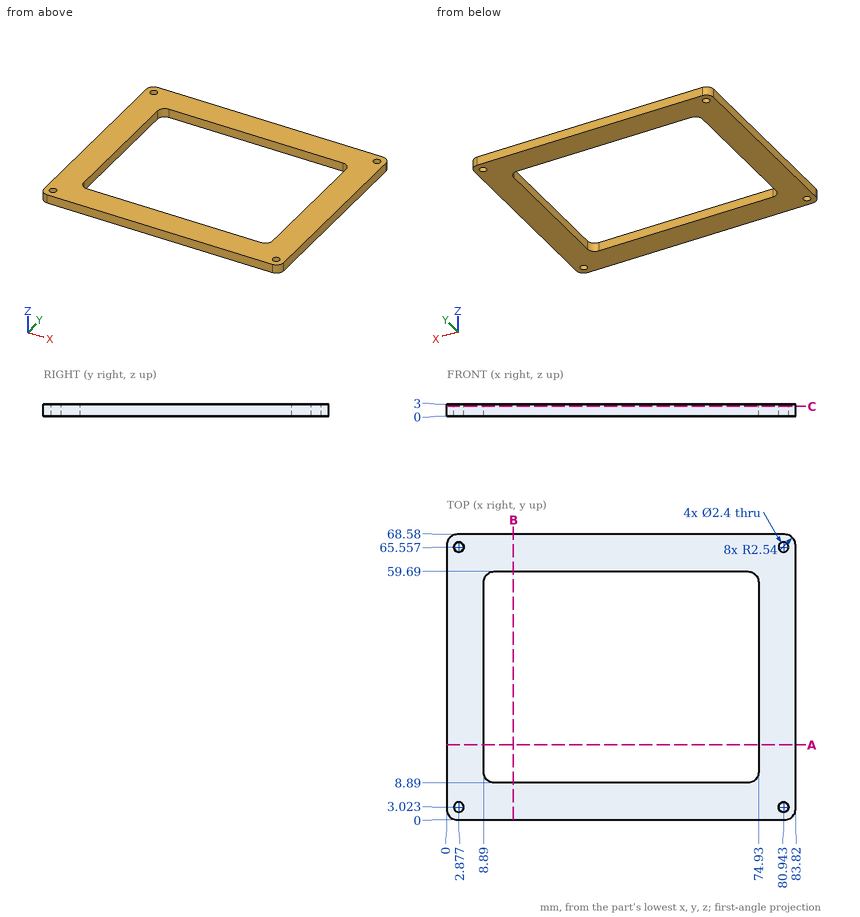
For this review, use the dimensioned drawing (mm, ordinates from the lowest corner) and the shaded views. Give positions to 0.01 mm unless a question says otherwise; leave off trailing zeros. Order: outer loops, then holes, each group sorted by start corner. A loop starts at its lowest first (then second) coordinate and runs counter-clockwise, first axis right, second up. Notation, with made-up numbers: M -21,44 L 32,44 A13 ccw 32,67 Z; hole C 18.5,-11.5 d1. An arc over 180 degrees is marked long. One line per question, with ' | ' between items. Start each with the question number.
1) Consider section C-C, the plane z = 2.4. Give the boundary of the cut face in (x, y).
2) Consider section B-B, the plane x = 16. Give the boundary of the cut face in (y, z).
3) Wall thickness on L1, parallel to X at y = 24.5, z = 2.8; L2, parallel to Y at x = 46, z = 1.4; L3, parallel to X at y = 64.5, z = 1.75 (1 decimal): over which ranges is each line inside the solid? List them lowest first. Write a range as from..to.
4) Consider section A-A, the plane y = 18. Give the boundary of the cut face in (x, z).
5) Clearance check with a flat-ended pin moving along its axis: P1, Ø2, axis at x = 80.94, y = 65.56, coming from the -Z side. State where the tip first meets the part, or that it passes through.
Found:
1) outline: M 0,2.54 A2.54 ccw 2.54,0 L 81.28,0 A2.54 ccw 83.82,2.54 L 83.82,66.04 A2.54 ccw 81.28,68.58 L 2.54,68.58 A2.54 ccw 0,66.04 Z; hole C 2.88,3.02 d2.4; hole C 2.88,65.56 d2.4; hole M 8.89,11.43 A2.54 ccw 11.43,8.89 L 72.39,8.89 A2.54 ccw 74.93,11.43 L 74.93,57.15 A2.54 ccw 72.39,59.69 L 11.43,59.69 A2.54 ccw 8.89,57.15 Z; hole C 80.94,3.02 d2.4; hole C 80.94,65.56 d2.4
2) outline: M 0,0 L 8.89,0 L 8.89,3 L 0,3 Z; M 59.69,0 L 68.58,0 L 68.58,3 L 59.69,3 Z
3) L1: x = 0..8.89, 74.93..83.82 | L2: y = 0..8.89, 59.69..68.58 | L3: x = 0..2.3, 3.4..80.4, 81.5..83.8
4) outline: M 0,0 L 8.89,0 L 8.89,3 L 0,3 Z; M 74.93,0 L 83.82,0 L 83.82,3 L 74.93,3 Z
5) P1: passes through
